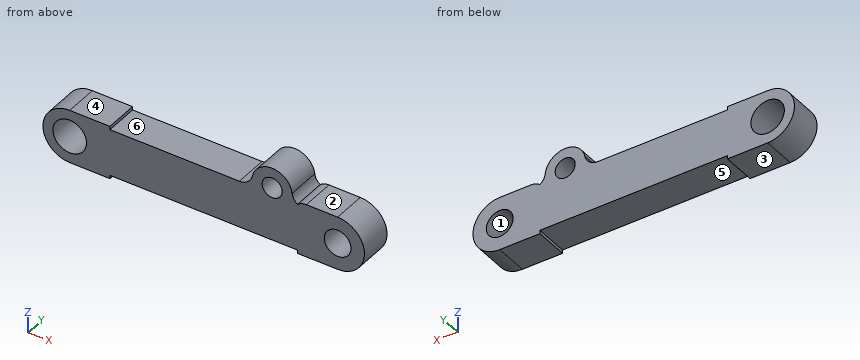
from build123d import *

# Parameters (mm, degrees)
SKETCH1_R           = 30
SKETCH1_R_2         = 50
SKETCH1_R_3         = 40
BOSS_EXTRUDE1_DEPTH = 100
FILLET1_R           = 40
FILLET2_R           = 40
FILLET3_R           = 40


with BuildPart() as part:
    # Sketch1 → Boss-Extrude1 (new body)
    with BuildSketch(Plane(origin=(0, 0, 0), x_dir=(1, 0, 0), z_dir=(0, 1, 0))):
        with BuildLine():
            Line((0, 80), (120, 80))
            Line((120, 80), (120, 70))
            Line((120, 70), (680, 70))
            Line((680, 70), (680, 80))
            Line((680, 80), (800, 80))
            ThreePointArc((800, 80), (880, 0), (800, -80))
            Line((800, -80), (680, -80))
            Line((680, -80), (680, -70))
            Line((680, -70), (661.048491655, -70))
            ThreePointArc((661.048491655, -70), (604.479949161, -150), (547.911406666, -70))
            Line((547.911406666, -70), (120, -70))
            Line((120, -70), (120, -80))
            Line((120, -80), (0, -80))
            ThreePointArc((0, -80), (-80, 0), (0, 80))
        make_face()
        with Locations(Location((604.479949161, -90, 0), (0, 0, 270))):
            Circle(SKETCH1_R, mode=Mode.SUBTRACT)
        with Locations(Location((0, 0, 0), (0, 0, 270))):
            Circle(SKETCH1_R_2, mode=Mode.SUBTRACT)
        with Locations(Location((800, 0, 0), (0, 0, 270))):
            Circle(SKETCH1_R_3, mode=Mode.SUBTRACT)
    extrude(amount=BOSS_EXTRUDE1_DEPTH)

    # Fillet1
    fillet1_edges = [part.edges().sort_by_distance(p)[0] for p in [
        (547.911406666, 50, 70),
    ]]
    fillet(fillet1_edges, radius=FILLET1_R)

    # Fillet2
    # the kernel refuses this fillet: 40 mm, written as the material it adds along each edge
    with BuildSketch(Plane(origin=(661.048491655, 0, 70), x_dir=(0.10855976910838376, 0, 0.9940899237650156), z_dir=(0, 1, 0))) as fillet2_piece_1:
        with BuildLine():
            CenterArc((36.641948169, 38.936942319), FILLET2_R, 210.161293822, 46.599784771)
            Line((2.05737137, 18.839503485), (1.365679834, 18.437554709))
            ThreePointArc((1.365679834, 18.437554709), (0.233413746, 9.506599558), (-0.795271939, 0.086847815))
            Line((-0.795271939, 0.086847815), (0.183209741, -0.778738846))
            ThreePointArc((0.183209741, -0.778738846), (13.740730563, 0.794586522), (27.298251386, -0.778738846))
            Line((27.298251386, -0.778738846), (27.481461127, 0))
        make_face()
    extrude(amount=100)

    # Fillet3
    # the kernel refuses this fillet: 40 mm, written as the material it takes off along each edge
    with BuildSketch(Plane(origin=(680, -66.143782777, 80), x_dir=(0, 0, -1), z_dir=(0, 1, 0))) as fillet3_piece_1:
        with BuildLine():
            CenterArc((40, -26.457513111), FILLET3_R, 138.590377891, 41.409622109)
            Line((0, -26.457513111), (-0.8, -26.457513111))
            Line((-0.8, -26.457513111), (-0.8, 0))
            Line((-0.8, 0), (0, 0.8))
            ThreePointArc((0, 0.8), (5, 0.8), (9.4, 0.529150262))
            Line((9.4, 0.529150262), (10, 0))
        make_face()
    extrude(amount=232.287565553, mode=Mode.SUBTRACT)


solid = part.part
For this review, take the finished solid that the model builds, in its own axes (mm). Face numbers are marked on the shaded views. A direction names the side the tool comes from. Round coordinates to 2 decimals unless told otherwise and drop trailing zeros. Write each loop counter-clockwise with the first axis right and the second up, starting at its lowest first coordinate (ties: lowest second). Pieces come first, ordered by that corner, then holes. Notation, with made-up numbers: (-30, 82.5) - (1, 82.5) arc R27 ccw to (1, 112.5) - close; hole circle Ø2 at (-29.75, -39). An arc over 180 degrees is marked (long way). Write item = value, one per line. Start each with the question number.
1. Consider section D-D on y = 67. State the section outline as (x, z) points.
2. Consider section C-C on x = -17. State the section outline as (y, z) points.
3. For pin 1 Ø3 at (x, y) = (550.5, 88) entering from -Z; pin 2 Ø6 at (x, y) = (598.5, 44.5) entering from +Z; pin 3 Ø5 at (x, y) = (537, 88.5) entering from +Z; pin 4 Ø8 at (x, z) = (603, -47.5) entering from -Y, all flat-tipped, find the tip position at first contact; note any pin that passes through.
4. Wall thickness on L1, parallel to X at y = 77.5, z = 0; L2, parallel to X at y = 71, z = 35.5; L3, parallel to Z at x = 242.5, y = 46: over which ranges is each line inside the solid? List them lowest first.
5. Draft analysis for pull direction Z (two halves, no side actions). For the marked faces 1, 2 and 3, state which applies: released by +Z, released by -Z, zero draft, split by the parting line, or undercut.
6. Consider section A-A on z = 0. State the section outline as (x, y) points.
7. Consider section B-B on z = 89. State the section outline as (x, y) points.
8. For the marked faces 4, 5 and 6, list the 3-axis set-ups (+Z, -Z, +X, -X, +Y, -Y) from which the entire face can be reached by the end or side of a thin tool; tool diameter is ignored.
Evaluation:
q1.outline = (0, -80) - (120, -80) - (120, -70) - (680, -70) - (680, -80) - (800, -80) arc R80 ccw to (800, 80) - (706.46, 80) arc R40 ccw to (680, 70) arc R40 cw to (664.03, 97.32) arc R60 ccw to (545.69, 102) arc R40 cw to (506.5, 70) - (120, 70) - (120, 80) - (0, 80) arc R80 ccw to start; hole circle Ø100 at (0, 0); hole circle Ø60 at (604.48, 90); hole circle Ø80 at (800, 0)
q2.outline = (0, -78.17) - (100, -78.17) - (100, -47.02) - (0, -47.02) - close; (0, 47.02) - (100, 47.02) - (100, 78.17) - (0, 78.17) - close
q3.pin_1 = -70
q3.pin_2 = 149.93
q3.pin_3 = 87.39
q3.pin_4 = 0
q4.L1 = -80 to -50, 50 to 760, 840 to 880
q4.L2 = -71.69 to -35.21, 35.21 to 781.57, 818.43 to 871.69
q4.L3 = -70 to 70
q5.face_1 = undercut
q5.face_2 = released by +Z
q5.face_3 = released by -Z
q6.outline = (-80, 0) - (-50, 0) - (-50, 100) - (-80, 100) - close; (50, 0) - (760, 0) - (760, 100) - (50, 100) - close; (840, 0) - (880, 0) - (880, 100) - (840, 100) - close
q7.outline = (540.54, 0) - (574.5, 0) - (574.5, 100) - (540.54, 100) - close; (634.46, 0) - (665.97, 0) - (665.97, 100) - (634.46, 100) - close
q8.face_4 = +Z, -X, +Y, -Y
q8.face_5 = -Z, +Y, -Y
q8.face_6 = +Z, +Y, -Y
